Check sheet for the modelled part. Datum: model origin and axes. Units: mm. A direction names the side the tool comes from. Round coordinates to 2 decimals unless told otherwise and drop trailing zeros. Loops run counter-clockwise (first coordinate to the right, second up) from the corner with the lowest first, then second, coordinate; pieces in that order, holes last. Notation, with made-up numbers: (43, -37.75) - (74, -37.75) arc R24 cw to (74, -6.75) - close; hole circle Ø6 at (33.5, 74). An arc over 180 degrees is marked (long way). Return JSON: item names as keys, results as strings.
from build123d import *

# Parameters (mm, degrees)
BOX_W             = 10
BOX_H             = 10
BOX_DEPTH         = 10
CYLINDER001_R     = 10
CYLINDER001_DEPTH = 5
CYLINDER002_R     = 3
CYLINDER002_DEPTH = 12
CYLINDER_R        = 18.5
CYLINDER_DEPTH    = 35


with BuildPart() as cube:
    # Box → Box (new body)
    with BuildSketch(Plane(origin=(2, -5, 7), x_dir=(1, 0, 0), z_dir=(0, 0, 1))):
        with Locations((5, 5)):
            Rectangle(BOX_W, BOX_H)
    extrude(amount=BOX_DEPTH)


with BuildPart() as cylinder001:
    # Cylinder001 → Cylinder001 (new body)
    with BuildSketch(Plane.XY):
        Circle(CYLINDER001_R)
    extrude(amount=CYLINDER001_DEPTH)


with BuildPart() as cylinder002:
    # Cylinder002 → Cylinder002 (new body)
    with BuildSketch(Plane.XY.offset(5)):
        Circle(CYLINDER002_R)
    extrude(amount=CYLINDER002_DEPTH)


with BuildPart() as cut:
    # Cylinder → Cylinder (new body)
    with BuildSketch(Plane.XY.offset(-35)):
        Circle(CYLINDER_R)
    extrude(amount=CYLINDER_DEPTH)

    # Fusion: union Cylinder001, Cylinder002
    add(cylinder001.part)
    add(cylinder002.part)

    # Cut: cut Cube
    add(cube.part, mode=Mode.SUBTRACT)


solid = cut.part
Q1. Sectioned sample at D-D (x = 6). Enter the section's corners in (y, z).
Answer key:
{"outline": "(-17.5, -35) - (17.5, -35) - (17.5, 0) - (8, 0) - (8, 5) - (-8, 5) - (-8, 0) - (-17.5, 0) - close"}
Q2. Tool access check on faces 1 (the face through (-2.17, -9.76, 2.46)), 2 (the face through (-1, 0, 17)), 3 (the face through (2, 0, 12)). Record the directions out of +Z, -Z, +X, -X, +Y, -Y that give a thin tool (end or side, any length) a straight path to the whole face; none if there is none.
Answer key:
{"face 1": "+Z", "face 2": "+Z, +X, -X, +Y, -Y", "face 3": "+Z, +X, +Y, -Y"}
Q3. Sectioned sample at A-A (x = 0). Enter the section's corners in (y, z).
Answer key:
{"outline": "(-18.5, -35) - (18.5, -35) - (18.5, 0) - (10, 0) - (10, 5) - (3, 5) - (3, 17) - (-3, 17) - (-3, 5) - (-10, 5) - (-10, 0) - (-18.5, 0) - close"}
Q4. Sectioned sample at B-B (y = 0). Enter the section's corners in (x, z), plus the area to 3 significant figures.
Answer key:
{"outline": "(-18.5, -35) - (18.5, -35) - (18.5, 0) - (10, 0) - (10, 5) - (3, 5) - (3, 7) - (2, 7) - (2, 17) - (-3, 17) - (-3, 5) - (-10, 5) - (-10, 0) - (-18.5, 0) - close", "area": "1,460 mm²"}
Q5. Depth check by flat-ended pin: P1, Ø11, axis at x = 5, y = 3, coming from the +Z side; P2, Ø1, axis at x = -3.5, z = 4, coming from the -Y side; P3, Ø3, axis at y = 12, z = -26.5, coming from the -X side; P4, Ø2, axis at y = 6, z = -11.5, coming from the -X side. Enter the tip coordinate at first touch or a pass-through.
Answer key:
{"P1": "stops at z = 17", "P2": "stops at y = -9.54", "P3": "stops at x = -15.23", "P4": "stops at x = -17.81"}
Q6. Sectioned sample at C-C (z = -13). Enter the section's corners in (x, y), plus the area to 3 significant figures.
Answer key:
{"outline": "circle Ø37 at (0, 0)", "area": "1,080 mm²"}
Q7. Scan lines: probe 1 along Z at (x, y) = (15.5, -10); probe 2 along Z at (x, y) = (-8.5, 2.5); probe 3 along Y at (x, z) = (9, 2). Record each from-to range of solid material in increasing order. Write a range as [from, to].
Answer key:
{"probe 1": "z = [-35, 0]", "probe 2": "z = [-35, 5]", "probe 3": "y = [-4.36, 4.36]"}
Q8. Draft check along Y on faces 4 (the face through (-4.01, -18.06, -17.74)), 5 (the face through (0, 0, -35)). Enter one of: released by +Y, released by -Y, zero draft, split by the parting line, or undercut.
Answer key:
{"face 4": "split by the parting line", "face 5": "zero draft"}
